Autodesk Inventor part; units mm, degrees
ref_plane "YZ Plane" through (0, 0, 0) normal (1, 0, 0) x (0, 1, 0)
ref_plane "XZ Plane" through (0, 0, 0) normal (0, 1, 0) x (-1, 0, 0)
ref_plane "XY Plane" through (0, 0, 0) normal (0, 0, 1) x (1, 0, 0)
sketch "Эскиз1" plane through (0, 0, 0) normal (0, 1, 0) x (-1, 0, 0)
  line L0 (0, 0) -> (12.5, 0)
  line L1 (12.5, 0) -> (12.5, 7.5)
  line L2 (12.5, 7.5) -> (0, 7.5)
  line L3 (0, 7.5) -> (0, 0)
  dimension "d0" = 12.5
  dimension "d1" = 7.5
extrude "Выдавливание1" add sketch "Эскиз1" along normal blind 10
sketch "Эскиз2" plane through (0, 0, 0) normal (0, -1, 0) x (1, 0, 0)
  line L0 (-1.42, 0.96) -> (-0.92, 0.96)
  line L1 (-0.92, 0.96) -> (-0.92, 1.46)
  line L2 (-0.92, 1.46) -> (-1.42, 1.46)
  line L3 (-1.42, 1.46) -> (-1.42, 0.96)
  line L4 (0, 0) -> (-12.5, 0)
  line L5 (0, 7.5) -> (0, 0)
  line L6 (-3.96, 0.96) -> (-3.46, 0.96)
  line L7 (-3.46, 0.96) -> (-3.46, 1.46)
  line L8 (-3.46, 1.46) -> (-3.96, 1.46)
  line L9 (-3.96, 1.46) -> (-3.96, 0.96)
  line L10 (-1.42, 6.04) -> (-0.92, 6.04)
  line L11 (-0.92, 6.04) -> (-0.92, 6.54)
  line L12 (-0.92, 6.54) -> (-1.42, 6.54)
  line L13 (-1.42, 6.54) -> (-1.42, 6.04)
  line L14 (-3.96, 6.04) -> (-3.46, 6.04)
  line L15 (-3.46, 6.04) -> (-3.46, 6.54)
  line L16 (-3.46, 6.54) -> (-3.96, 6.54)
  line L17 (-3.96, 6.54) -> (-3.96, 6.04)
  line L18 (-11.58, 6.04) -> (-11.08, 6.04)
  line L19 (-11.08, 6.54) -> (-11.58, 6.54)
  line L20 (-11.58, 6.54) -> (-11.58, 6.04)
  line L21 (-11.08, 6.04) -> (-11.08, 6.54)
  line L22 (-11.08, 1.46) -> (-11.58, 1.46)
  line L23 (-11.08, 0.96) -> (-11.08, 1.46)
  line L24 (-11.58, 1.46) -> (-11.58, 0.96)
  line L25 (-11.58, 0.96) -> (-11.08, 0.96)
  dimension "d4" = 0.5
  dimension "d5" = 0.5
  dimension "d7" = 0.96
  dimension "d8" = 0.92
  dimension "d11" = 2.54
  dimension "d14" = 5.08
  dimension "d19" = 7.62
extrude "Выдавливание2" add sketch "Эскиз2" along normal blind 3.5
fillet "Сопряжение1" radius 0.3 8 edges at (-6.25, 10, 0) (-12.5, 10, 3.75) (-6.25, 10, 7.5) (0, 10, 3.75) (0, 5, 7.5) (0, 5, 0) (-12.5, 5, 0) (-12.5, 5, 7.5)
properties part number "NRP03K"
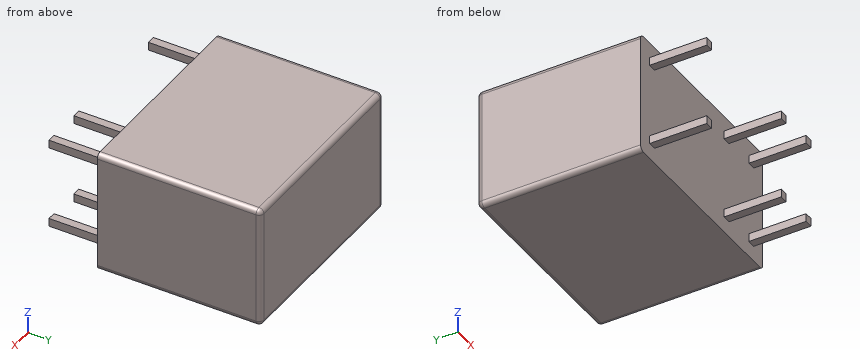
Input: part model. Units: mm. Frame: model coordinates. Give positions to 0.01 mm unless a question says otherwise; leave off trailing zeros. Write each loop counter-clockwise with the first axis right and the second up, starting at its lowest first coordinate (ties: lowest second). Pieces come first, ordered by that corner, then holes.
Q1. Material intervals for probe 1 along Z at (x, y) = (-3.5, -2.5); probe 2 along X at (y, z) = (-2, 6.5); probe 3 along Y at (x, z) = (-6.5, 4.75), sorted ascending.
Q2. First-contact query: P1, Ø0.6, axis at x = -4, y = -1.5, coming from the +Z side; P2, Ø2, axis at x = -9, z = 2, coming from the -Y side; P3, Ø0.6, axis at y = -2.5, z = 6.5, coming from the +X side. Flat tips, straight axial feed; report the tip coordinate or a pass-through.
Q3. Section A-A, the plane x = -10. Output: boundary loops of the cut face in (y, z), plus the area to 3 significant figures.
Q4. Section B-B, the plane z = 3.25. Output: boundary loops of the cut face in (x, y).
Filled in:
1. probe 1: z = 0.96 to 1.46, 6.04 to 6.54
1. probe 2: x = -11.58 to -11.08, -3.96 to -3.46, -1.42 to -0.92
1. probe 3: y = 0 to 10
2. P1: stops at z = 6.54
2. P2: stops at y = 0
2. P3: stops at x = -0.92
3. outline: (0, 0) - (9.7, 0) arc R0.3 ccw to (10, 0.3) - (10, 7.2) arc R0.3 ccw to (9.7, 7.5) - (0, 7.5) - close
3. area: 75.0 mm2
4. outline: (-12.5, 0) - (0, 0) - (0, 9.7) arc R0.3 ccw to (-0.3, 10) - (-12.2, 10) arc R0.3 ccw to (-12.5, 9.7) - close
